Here's how the part is built. I have some questions about the finished solid (model axes, mm). Give positions to 0.01 mm unless a question says otherwise; leave off trailing zeros. Write each loop counter-clockwise with the first axis right and the second up, starting at its lowest first coordinate (ties: lowest second). Pieces come first, ordered by that corner, then holes. Notation, with made-up numbers: (44.25, 15.25) -> (80.25, 15.25) arc R8 ccw to (80.25, 21.25) -> close; hole circle Ø8 at (81.25, 31.5). An arc over 180 degrees is marked (long way). Return JSON: item names as keys, results as strings.
Autodesk Inventor part; units mm, degrees
ref_plane "YZ Plane" through (0, 0, 0) normal (1, 0, 0) x (0, 1, 0)
ref_plane "XZ Plane" through (0, 0, 0) normal (0, 1, 0) x (-1, 0, 0)
ref_plane "XY Plane" through (0, 0, 0) normal (0, 0, 1) x (1, 0, 0)
sketch "スケッチ1" plane through (0, 0, 0) normal (0, 0, 1) x (1, 0, 0)
  line L0 (-5, -35.5) -> (5, -35.5)
  line L1 (5, -35.5) -> (5, 35.5)
  line L2 (5, 35.5) -> (-5, 35.5)
  line L3 (-5, 35.5) -> (-5, -35.5)
  line L4 (-5, -35.5) -> (5, 35.5) construction
  line L5 (5, -35.5) -> (-5, 35.5) construction
  line L6 (-5, -35.5) -> (100, -35.5)
  line L7 (100, -35.5) -> (100, -25.5)
  line L8 (100, -25.5) -> (-5, -25.5)
  line L9 (-5, -25.5) -> (-5, -35.5)
  line L10 (47.5, -35.5) -> (47.5, -45.5)
  arc A0 (-5, -25.5) -> (100, -25.5) centre (47.5, 107.3125) ccw
  arc A1 (-5, -35.5) -> (100, -35.5) centre (47.5, 97.3125) ccw
  point P0 (0, 0)
  point P1 (5, -29.0296)
  dimension "d0" = 10
  dimension "d1" = 71
  dimension "d2" = 105
  dimension "d3" = 10
  dimension "d4" = 10
extrude "押し出し1" add sketch "スケッチ1" along normal mid plane 2.5 contours L3 A0 L1 L0 | L0 L6 L10 A1 | L1 A0 L6 | L3 L2 L1 L8 | L8 L1 A0 | L10 L6 A1 | A0 L7 L6 picked at (-0.5654, -25.9196)
sketch "スケッチ2" plane through (0, 0, 1.25) normal (0, 0, 1) x (1, 0, 0)
  line L0 (5, 35.5) -> (-5, 35.5)
  line L1 (5, -29.0296) -> (5, 35.5)
  circle A0 centre (0, 30.5) radius 3.05
  circle A1 centre (0, 30.5) radius 3.65
  point P0 (0, 0)
  dimension "d7" = 5
  dimension "d8" = 5
  dimension "d9" = 6.1
  dimension "d10" = 7.3
extrude "押し出し2" cut sketch "スケッチ2" against normal blind 0.6 contours A0 | A1
sketch "スケッチ3" plane through (0, 30.5, 0.65) normal (0, 0, 1) x (1, 0, 0)
  circle A0 centre (0, 0) radius 3.05
  point P0 (0, -30.5)
  dimension "d13" = 6.1
extrude "押し出し3" cut sketch "スケッチ3" against normal blind 1.9
sketch "スケッチ6" plane through (0, 0, 1.25) normal (0, 0, 1) x (1, 0, 0)
  circle A0 centre (0, 30.5) radius 3.65
  line L0 (-5, 35.5) -> (-5, -35.5)
  arc A1 (-5, -35.5) -> (100, -35.5) centre (47.5, 97.3125) ccw
  line L1 (100, -35.5) -> (100, -25.5)
  arc A2 (5, -29.0296) -> (100, -25.5) centre (47.5, 107.3125) ccw
  line L2 (5, -29.0296) -> (5, 35.5)
  line L3 (5, 35.5) -> (-5, 35.5)
  circle A3 centre (0, 30.5) radius 5.65
  point P0 (0, 0)
  point P1 (-5, 27.8689)
  point P2 (-5, 33.1311)
  point P3 (-2.6311, 35.5)
  point P4 (2.6311, 35.5)
  point P5 (5, 33.1311)
  point P6 (5, 27.8689)
  dimension "d18" = 11.3
extrude "押し出し5" add sketch "スケッチ6" against normal blind 2.5 contours L0 A3 | A3 L3 | L2 A3
sketch "スケッチ7" plane through (0, 0, 1.25) normal (0, 0, 1) x (1, 0, 0)
  circle A0 centre (0, 30.5) radius 3.65
  line L0 (-5, 35.5) -> (-5, 33.1311)
  arc A1 (-5, 33.1311) -> (-5, 27.8689) centre (0, 30.5) ccw
  line L1 (-5, 27.8689) -> (-5, -35.5)
  arc A2 (-5, -35.5) -> (100, -35.5) centre (47.5, 97.3125) ccw
  line L2 (100, -35.5) -> (100, -25.5)
  arc A3 (5, -29.0296) -> (100, -25.5) centre (47.5, 107.3125) ccw
  line L3 (5, -29.0296) -> (5, 27.8689)
  arc A4 (5, 27.8689) -> (5, 33.1311) centre (0, 30.5) ccw
  line L4 (5, 33.1311) -> (5, 35.5)
  line L5 (5, 35.5) -> (2.6311, 35.5)
  arc A5 (2.6311, 35.5) -> (-2.6311, 35.5) centre (0, 30.5) ccw
  line L6 (-2.6311, 35.5) -> (-5, 35.5)
  circle A6 centre (0, 30.5) radius 5.65
  point P0 (0, 0)
  point P1 (-2.6311, 35.5)
  point P2 (2.6311, 35.5)
extrude "押し出し6" cut sketch "スケッチ7" against normal blind 2.5 contours L6 A6 L0 | L5 L4 A6
fillet "フィレット1" radius 2 4 edges at (-5, -35.5, 0) (5, -29.0296, 0) (100, -25.5, 0) (100, -35.5, 0)
properties part number "指_中"
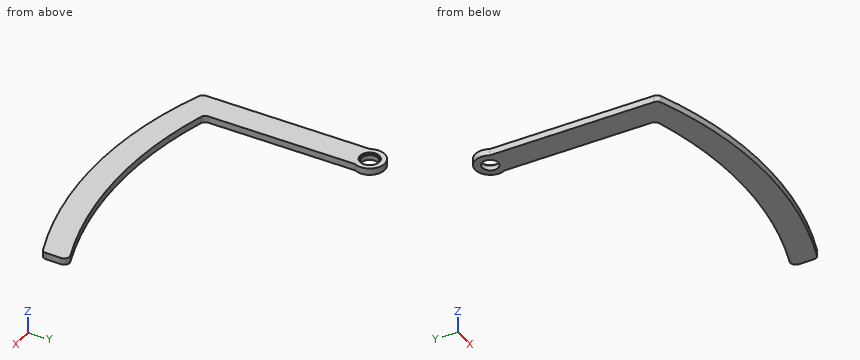
1. For pin 1 Ø1 at (x, z) = (65, -1) entering from -Y; pin 2 Ø4.5 at (x, y) = (0, 30.5) entering from -Z, each with a flat end and sliding along its axis, tell me the tip position at first contact or that it passes through.
Taken from the geometry:
{"pin 1": "stops at y = -44.48", "pin 2": "passes through"}
2. Suppose I cut it at B-B, the plane y = 30.5. List the corners of the cut face in (x, z) for me, and give its area (3 significant figures).
Taken from the geometry:
{"outline": "(-5.65, -1.25) -> (-3.05, -1.25) -> (-3.05, 0.65) -> (-3.65, 0.65) -> (-3.65, 1.25) -> (-5.65, 1.25) -> close; (3.05, -1.25) -> (5.65, -1.25) -> (5.65, 1.25) -> (3.65, 1.25) -> (3.65, 0.65) -> (3.05, 0.65) -> close", "area": "12.3 mm²"}
3. If I drill on line 1 (Y direction, x = 0, z = -0.45); line 2 (X direction, y = 10.5, z = 0.9); line 3 (Y direction, x = 89, z = 0.8), over which ranges is the centre line in solid material (lowest first)? Write a range as [from, to].
Taken from the geometry:
{"line 1": "y = [-37.37, 27.45], [33.55, 36.15]", "line 2": "x = [-5, 5]", "line 3": "y = [-39.34, -29.34]"}
4. Suppose I cut it at C-C, the plane x = 0. List the corners of the cut face in (y, z) for me.
Taken from the geometry:
{"outline": "(-37.37, -1.25) -> (27.45, -1.25) -> (27.45, 0.65) -> (26.85, 0.65) -> (26.85, 1.25) -> (-37.37, 1.25) -> close; (33.55, -1.25) -> (36.15, -1.25) -> (36.15, 1.25) -> (34.15, 1.25) -> (34.15, 0.65) -> (33.55, 0.65) -> close"}
5. Suppose I cut it at D-D, the plane y = -12. List the corners of the cut face in (x, z) for me, and give its area (3 significant figures).
Taken from the geometry:
{"outline": "(-5, -1.25) -> (5, -1.25) -> (5, 1.25) -> (-5, 1.25) -> close", "area": "25.0 mm²"}
